Model file for the job. Use its own axes, mm. A direction names the side the tool comes from. Give positions to 0.01 mm unless a question says otherwise; leave off trailing zeros. Order: outer loops, then holes, each group sorted by start corner. A loop starts at its lowest first (then second) coordinate and runs counter-clockwise, first axis right, second up. Notation, with made-up numbers: (80, -39.75) - (133, -39.75) arc R19 ccw to (133, -9.75) - close; hole circle Ø3 at (29, -36.5). An arc over 180 degrees is marked (long way). Return JSON: item names as keys, results as strings. Group by question number.
from build123d import *

# Parameters (mm, degrees)
CROQUIS2_W              = 31
CROQUIS2_H              = 12
SALIENTE_EXTRUIR1_DEPTH = 13
CROQUIS3_W              = 25.1
CROQUIS3_H              = 10.1
CORTAR_EXTRUIR1_DEPTH   = 9
CROQUIS6_W              = 1.1
CROQUIS6_H              = 9
CORTAR_EXTRUIR3_DEPTH   = 32
CROQUIS7_R              = 1.5
CORTAR_EXTRUIR4_DEPTH   = 14


with BuildPart() as part:
    # Croquis2 → Saliente-Extruir1 (new body)
    with BuildSketch(Plane.XY):
        Rectangle(CROQUIS2_W, CROQUIS2_H)
    extrude(amount=SALIENTE_EXTRUIR1_DEPTH)

    # Croquis3 → Cortar-Extruir1 (cut)
    with BuildSketch(Plane.XZ.offset(6)):
        with Locations((0, 7.95)):
            Rectangle(CROQUIS3_W, CROQUIS3_H)
    extrude(amount=-CORTAR_EXTRUIR1_DEPTH, mode=Mode.SUBTRACT)

    # Croquis6 → Cortar-Extruir3 (cut, through all)
    with BuildSketch(Plane.ZY.offset(15.5)):
        with Locations((3.45, -1.5)):
            Rectangle(CROQUIS6_W, CROQUIS6_H)
    extrude(amount=-CORTAR_EXTRUIR3_DEPTH, mode=Mode.SUBTRACT)

    # Croquis7 → Cortar-Extruir4 (cut, through all)
    with BuildSketch(Plane(origin=(0, 0, 0), x_dir=(-1, 0, 0), z_dir=(0, 0, -1))):
        with Locations((-8.4125, -2.05)):
            Circle(CROQUIS7_R)
        with Locations((8.4125, -2.05)):
            Circle(CROQUIS7_R)
    extrude(amount=-CORTAR_EXTRUIR4_DEPTH, mode=Mode.SUBTRACT)


solid = part.part
(1) Drill centre lines: L1, parallel to X at y = -5, z = 6.75; L2, parallel to Z at x = 4.5, y = -3; L3, parallel to Y at x = 7.5, z = 6.5. Where is each one in solid material? Low to high.
(2) Slice it at B-B (z = 8.25). Give the cut face in (x, y), and give its area (3 significant figures).
(3) Drop flat-ended pins along their axis: pin 1 Ø3 at (x, y) = (8, -4.5) entering from +Z; pin 2 Ø2.5 at (x, y) = (8.41, -2.05) entering from -Z. Give the stop position or say it passes through.
(4) Slice it at C-C (z = 1.75). Give the cut face in (x, y), and give its area (3 significant figures).
(5) Pull direction Z, two halves, no side cores. Call faces 4 (the face through (0, 0, 0)), 5 (the face through (0, -2, 2.9)), 6 (the face through (12.55, -2, 8)): released by +Z, released by -Z, zero draft, split by the parting line, or undercut.
(6) 3-axis set-ups, long thin cutter, end or side, ignore diameter. For faces 1 (the face through (14, -6, 8)), 2 (the face through (-12.55, -2, 8)), 3 (the face through (14, -2, 4)): which of +Z, -Z, +X, -X, +Y, -Y reach the whole face in a straight line?
(7) Slice it at A-A (y = -2.05). Give the cut face in (x, z), and give its area (3 significant figures).
(8) Slice it at D-D (x = -11). Give the cut face in (y, z).
Result set:
{
 "1": {"L1": "x = -15.5 to -12.55, 12.55 to 15.5", "L2": "z = 0 to 2.9", "L3": "y = 3 to 6"},
 "2": {"outline": "(-15.5, -6) - (-12.55, -6) - (-12.55, 3) - (12.55, 3) - (12.55, -6) - (15.5, -6) - (15.5, 6) - (-15.5, 6) - close", "area": "146 mm²"},
 "3": {"pin 1": "stops at z = 2.9", "pin 2": "passes through"},
 "4": {"outline": "(-15.5, -6) - (15.5, -6) - (15.5, 6) - (-15.5, 6) - close; hole circle Ø3 at (-8.41, -2.05); hole circle Ø3 at (8.41, -2.05)", "area": "358 mm²"},
 "5": {"face 4": "released by -Z", "face 5": "undercut", "face 6": "zero draft"},
 "6": {"face 1": "+Z, -Z, +X, -X, -Y", "face 2": "+Z, -Y", "face 3": "+X, -X, -Y"},
 "7": {"outline": "(-15.5, 0) - (-9.91, 0) - (-9.91, 2.9) - (-15.5, 2.9) - close; (-15.5, 4) - (-12.55, 4) - (-12.55, 13) - (-15.5, 13) - close; (-6.91, 0) - (6.91, 0) - (6.91, 2.9) - (-6.91, 2.9) - close; (9.91, 0) - (15.5, 0) - (15.5, 2.9) - (9.91, 2.9) - close; (12.55, 4) - (15.5, 4) - (15.5, 13) - (12.55, 13) - close", "area": "126 mm²"},
 "8": {"outline": "(-6, 0) - (6, 0) - (6, 13) - (3, 13) - (3, 2.9) - (-6, 2.9) - close"}
}
